Autodesk Inventor part; units mm, degrees
ref_plane "YZ Plane" through (0, 0, 0) normal (1, 0, 0) x (0, 1, 0)
ref_plane "XZ Plane" through (0, 0, 0) normal (0, 1, 0) x (-1, 0, 0)
ref_plane "XY Plane" through (0, 0, 0) normal (0, 0, 1) x (1, 0, 0)
sketch "Sketch1" plane through (0, 0, 0) normal (0, 1, 0) x (-1, 0, 0)
  line L0 (-2.5, 2.5) -> (2.5, 2.5)
  line L1 (2.5, 2.5) -> (2.5, -2.5)
  line L2 (2.5, -2.5) -> (-2.5, -2.5)
  line L3 (-2.5, -2.5) -> (-2.5, 2.5)
  line L4 (-2.5, 2.5) -> (2.5, -2.5) construction
  line L5 (2.5, 2.5) -> (-2.5, -2.5) construction
  point P0 (0, 0)
  dimension "d0" = 5
  dimension "d1" = 5
extrude "Extrusion1" add sketch "Sketch1" along normal blind 8
shell "Shell1" thickness 1 removed faces 1 at (-0.8333, 8, -0.8333)
sketch "Sketch9" plane through (2.5, 0, 2.5) normal (1, 0, 0) x (0, 0, -1)
  line L0 (1.5, 6.5) -> (3.5, 6.5)
  line L1 (3.5, 6.5) -> (3.5, 7.5)
  line L2 (3.5, 7.5) -> (1.5, 7.5)
  line L3 (1.5, 7.5) -> (1.5, 6.5)
  line L4 (1.5, 6.5) -> (3.5, 7.5) construction
  line L5 (3.5, 6.5) -> (1.5, 7.5) construction
  line L6 (0, 8) -> (5, 8)
  point P0 (2.5, 0)
  point P1 (2.5, 7)
  dimension "d10" = 1
  dimension "d14" = 2
  dimension "d15" = 1
extrude "Extrusion4" add sketch "Sketch9" along normal blind 0.5 draft -30
sketch "Sketch10" plane through (-2.5, 0, -2.5) normal (-1, 0, 0) x (0, 0, 1)
  line L0 (1.5, 6.5) -> (3.5, 6.5)
  line L1 (3.5, 6.5) -> (3.5, 7.5)
  line L2 (3.5, 7.5) -> (1.5, 7.5)
  line L3 (1.5, 7.5) -> (1.5, 6.5)
  line L4 (1.5, 6.5) -> (3.5, 7.5) construction
  line L5 (3.5, 6.5) -> (1.5, 7.5) construction
  line L6 (0, 8) -> (5, 8)
  point P0 (2.5, 0)
  point P1 (2.5, 7)
  dimension "d13" = 1
  dimension "d16" = 2
  dimension "d17" = 1
extrude "Extrusion5" add sketch "Sketch10" along normal blind 0.5 draft -30
sketch "Sketch11" plane through (2.5, 0, -2.5) normal (0, 0, -1) x (-1, 0, 0)
  line L0 (2.5, 7.862) -> (2.5, 3.6245) construction
  line L1 (1.5, 7.862) -> (1.5, 3.6245)
  line L2 (3.5, 3.6245) -> (3.5, 7.862)
  arc A0 (3.5, 7.862) -> (1.5, 7.862) centre (2.5, 7.862) ccw
  arc A1 (1.5, 3.6245) -> (3.5, 3.6245) centre (2.5, 3.6245) ccw
  point P0 (2.5, 0)
  point P1 (2.5, 5.7432)
  dimension "d20" = 2
extrude "Extrusion6" cut sketch "Sketch11" against normal through all
sketch "Sketch12" plane through (2.5, 0, -2.5) normal (0, 0, -1) x (-1, 0, 0)
  line L0 (1.5, 7.862) -> (1.5, 3.6245)
  line L1 (1.5, 7.862) -> (3.5, 7.862)
  line L2 (3.5, 7.862) -> (3.5, 10.4679)
  line L3 (3.5, 10.4679) -> (1.5, 10.4679)
  line L4 (1.5, 10.4679) -> (1.5, 7.862)
  point P0 (2.5, 0)
  dimension "d23" = 2
extrude "Extrusion7" cut sketch "Sketch12" against normal through all
equation "\"d16\" = d14"
equation "\"d17\" = d15"
properties part number "snapfit_part_v02"
Part model, mm, in its own coordinate system. A direction names the side the tool comes from. Coordinates: 2 decimals unless noted, no trailing zeros. Write each loop counter-clockwise with the first axis right and the second up, starting at its lowest first coordinate (ties: lowest second). Pieces come first, ordered by that corner, then holes. Notation, with made-up numbers: (38, 81) - (78, 81) arc R13 cw to (78, 89) - close; hole circle Ø4 at (25.5, -8). An arc over 180 degrees is marked (long way). Put each result on its own line as item: value.
1. Band-saw the part on C-C (z = -1.15). Write the cut outline in (x, y), then the cut area to 3 significant figures.
Final values:
outline: (-2.5, 0) - (2.5, 0) - (2.5, 8) - (1.5, 8) - (1.5, 1) - (-1.5, 1) - (-1.5, 8) - (-2.5, 8) - close
area: 19.0 mm²
2. Band-saw the part on A-A (y = 2.5). Write the cut outline in (x, z), then the cut area to 3 significant figures.
Final values:
outline: (-2.5, -2.5) - (2.5, -2.5) - (2.5, 2.5) - (-2.5, 2.5) - close; hole (-1.5, -1.5) - (1.5, -1.5) - (1.5, 1.5) - (-1.5, 1.5) - close
area: 16.0 mm²
3. Probe line 1 along X through (y, z) = (5, 2); line 2 along X through (y, z) = (7.75, 1.15). List the from-to ranges inside material, lowest first. Write a range as [from, to].
Final values:
line 1: x = [-2.5, -1], [1, 2.5]
line 2: x = [-2.5, -1.5], [1.5, 2.5]
4. Two-plate mould, pull along X, no slides. Class faces 1 (the cylindrical face through (0.022, 2.625, -2.007)), 2 (the flat face through (2.5, 4, 0)), 3 (the flat face through (-1, 3, 2.5)), 4 (the flat face through (-1, 6, -2)): +X half, -X half, draft (parallel to the pull), parting line (faces both ways), or undercut.
Final values:
face 1: undercut
face 2: +X half
face 3: draft
face 4: undercut
5. Band-saw the part on B-B (y = 4.5). Write the cut outline in (x, z), then the cut area to 3 significant figures.
Final values:
outline: (-2.5, -2.5) - (-1, -2.5) - (-1, -1.5) - (-1.5, -1.5) - (-1.5, 1.5) - (-1, 1.5) - (-1, 2.5) - (-2.5, 2.5) - close; (1, -2.5) - (2.5, -2.5) - (2.5, 2.5) - (1, 2.5) - (1, 1.5) - (1.5, 1.5) - (1.5, -1.5) - (1, -1.5) - close
area: 12.0 mm²
6. Flat gauge pins, fed straight in: pin 1 Ø0.8 at (y, z) = (5.5, -2) entering from -X; pin 2 Ø0.8 at (y, z) = (5, 2) entering from +X; pin 3 Ø1.5 at (x, y) = (0, 3.5) entering from +Z (3 decimals). Where does each tip first touch, or does it go through?
Final values:
pin 1: stops at x = -2.5
pin 2: stops at x = 2.5
pin 3: passes through
7. Band-saw the part on D-D (x = 0). Write the cut outline in (y, z), then the cut area to 3 significant figures.
Final values:
outline: (0, -2.5) - (2.62, -2.5) - (2.62, -1.5) - (1, -1.5) - (1, 1.5) - (2.62, 1.5) - (2.62, 2.5) - (0, 2.5) - close
area: 8.25 mm²
8. 3-axis set-ups, long thin cutter, end or side, ignore diameter. For faces 5 (the flat face through (1, 3, -2.5)), 6 (the flat face through (1, 6, 2)), 7 (the flat face through (1.5, 4, 0)): which of +Z, -Z, +X, -X, +Y, -Y reach the whole face in a straight line?
Final values:
face 5: -Z, +X, -X, +Y, -Y
face 6: +Z, -Z, +Y
face 7: +Y
